```python
from build123d import *

# Parameters (mm, degrees)
ESQUISSE2_W                                      = 120
ESQUISSE2_H                                      = 90
BOSS_EXTRU_1_DEPTH                               = 2
ESQUISSE3_R                                      = 5
BOSS_EXTRU_2_DEPTH                               = 8
CHAMBRAGE_POUR_VIS_T_TE_RONDE_BOMB_E_D           = 3.7973
CHAMBRAGE_POUR_VIS_T_TE_RONDE_BOMB_E_CBORE_D     = 7.54126
CHAMBRAGE_POUR_VIS_T_TE_RONDE_BOMB_E_CBORE_DEPTH = 2.4638
R_P_TITION_LIN_AIRE1_COUNT                       = 2
R_P_TITION_LIN_AIRE1_PITCH                       = 96
R_P_TITION_LIN_AIRE1_COUNT_DIR2                  = 2
R_P_TITION_LIN_AIRE1_PITCH_DIR2                  = 66
ENL_V_MAT_EXTRU_1_DEPTH                          = 8
R_P_TITION_LIN_AIRE2_COUNT                       = 5
R_P_TITION_LIN_AIRE2_PITCH                       = 9
R_P_TITION_LIN_AIRE2_COL_COUNT                   = 5
R_P_TITION_LIN_AIRE2_COL_PITCH                   = 9
ESQUISSE8_W                                      = 120
ESQUISSE8_H                                      = 90
ESQUISSE8_W_2                                    = 116
ESQUISSE8_H_2                                    = 86
BOSS_EXTRU_3_DEPTH                               = 25
ENL_V_MAT_EXTRU_2_REACH                          = 132.973
ENL_V_MAT_EXTRU_3_DEPTH                          = 2
CONG_1_R                                         = 3


with BuildPart() as part:
    # Esquisse2 → Boss.-Extru.1 (new body)
    with BuildSketch(Plane.XY):
        Rectangle(ESQUISSE2_W, ESQUISSE2_H)
    extrude(amount=BOSS_EXTRU_1_DEPTH)

    # Esquisse3 → Boss.-Extru.2 (add)
    with BuildSketch(Plane.XY.offset(2)):
        with Locations((-48, 33)):
            Circle(ESQUISSE3_R)
        with Locations((48, 33)):
            Circle(ESQUISSE3_R)
        with Locations((48, -33)):
            Circle(ESQUISSE3_R)
        with Locations((-48, -33)):
            Circle(ESQUISSE3_R)
    extrude(amount=BOSS_EXTRU_2_DEPTH)

    # Chambrage pour vis à tête ronde bombée #61 (through all)
    with Locations(Plane(origin=(0, 0, 0), x_dir=(-1, 0, 0), z_dir=(0, 0, -1))):
        with Locations((48, -33)):
            chambrage_pour_vis_t_te_ronde_bomb_e = CounterBoreHole(CHAMBRAGE_POUR_VIS_T_TE_RONDE_BOMB_E_D / 2, CHAMBRAGE_POUR_VIS_T_TE_RONDE_BOMB_E_CBORE_D / 2, CHAMBRAGE_POUR_VIS_T_TE_RONDE_BOMB_E_CBORE_DEPTH)

    # Répétition linéaire1: Chambrage pour vis _ t_te ronde bomb_e 2 × 2
    with Locations(*[(i * R_P_TITION_LIN_AIRE1_PITCH, j * R_P_TITION_LIN_AIRE1_PITCH_DIR2, 0) for i in range(R_P_TITION_LIN_AIRE1_COUNT) for j in range(R_P_TITION_LIN_AIRE1_COUNT_DIR2) if (i, j) != (0, 0)]):
        add(chambrage_pour_vis_t_te_ronde_bomb_e, mode=Mode.SUBTRACT)

    # Esquisse7 → Enlèv. mat.-Extru.1 (cut)
    with BuildSketch(Plane.XY.offset(2)):
        with BuildLine():
            Line((-1.5, -30), (-1.5, 30))
            ThreePointArc((-1.5, 30), (0, 31.5), (1.5, 30))
            Line((1.5, 30), (1.5, -30))
            ThreePointArc((1.5, -30), (0, -31.5), (-1.5, -30))
        make_face()
    enl_v_mat_extru_1 = extrude(amount=-ENL_V_MAT_EXTRU_1_DEPTH, mode=Mode.SUBTRACT)

    # Répétition linéaire2: Enlèv. mat.-Extru.1 ×5
    with Locations(*[(-i * R_P_TITION_LIN_AIRE2_PITCH, 0, 0) for i in range(1, R_P_TITION_LIN_AIRE2_COUNT)]):
        add(enl_v_mat_extru_1, mode=Mode.SUBTRACT)

    # Répétition linéaire2 col: Enlèv. mat.-Extru.1 ×5
    with Locations(*[(i * R_P_TITION_LIN_AIRE2_COL_PITCH, 0, 0) for i in range(1, R_P_TITION_LIN_AIRE2_COL_COUNT)]):
        add(enl_v_mat_extru_1, mode=Mode.SUBTRACT)

    # Esquisse8 → Boss.-Extru.3 (add)
    with BuildSketch(Plane.XY.offset(2)):
        Rectangle(ESQUISSE8_W, ESQUISSE8_H)
        Rectangle(ESQUISSE8_W_2, ESQUISSE8_H_2, mode=Mode.SUBTRACT)
    extrude(amount=BOSS_EXTRU_3_DEPTH)

    # Esquisse9 → Enlèv. mat.-Extru.2 (cut, up to next)
    with BuildSketch(Plane.ZY.offset(60), mode=Mode.PRIVATE) as enl_v_mat_extru_2_sk1:
        with BuildLine():
            Line((23, 0.689181082), (23, -29.310818918))
            ThreePointArc((23, -29.310818918), (18, -34.310818918), (13, -29.310818918))
            Line((13, -29.310818918), (13, 0.689181082))
            ThreePointArc((13, 0.689181082), (18, 5.689181082), (23, 0.689181082))
        make_face()
    enl_v_mat_extru_2_tool1 = extrude(enl_v_mat_extru_2_sk1.sketch, amount=-ENL_V_MAT_EXTRU_2_REACH, mode=Mode.PRIVATE) & part.part
    add(enl_v_mat_extru_2_tool1.solids().sort_by_distance((-60, -14.310819, 18))[0], mode=Mode.SUBTRACT)

    # Esquisse10 → Enlèv. mat.-Extru.3 (cut)
    with BuildSketch(Plane(origin=(60, 0, 0), x_dir=(0, 0, -1), z_dir=(1, 0, 0))):
        with BuildLine():
            Line((-20, -8.249494847), (-20, 6.750505153))
            ThreePointArc((-20, 6.750505153), (-15, 11.750505153), (-10, 6.750505153))
            Line((-10, 6.750505153), (-10, -8.249494847))
            ThreePointArc((-10, -8.249494847), (-15, -13.249494847), (-20, -8.249494847))
        make_face()
    extrude(amount=-ENL_V_MAT_EXTRU_3_DEPTH, mode=Mode.SUBTRACT)

    # Congé1
    cong_1_edges = [part.edges().sort_by_distance(p)[0] for p in [
        (-60, 45, 13.5),
        (60, 45, 13.5),
        (60, -45, 13.5),
        (-60, -45, 13.5),
    ]]
    fillet(cong_1_edges, radius=CONG_1_R)


solid = part.part
```
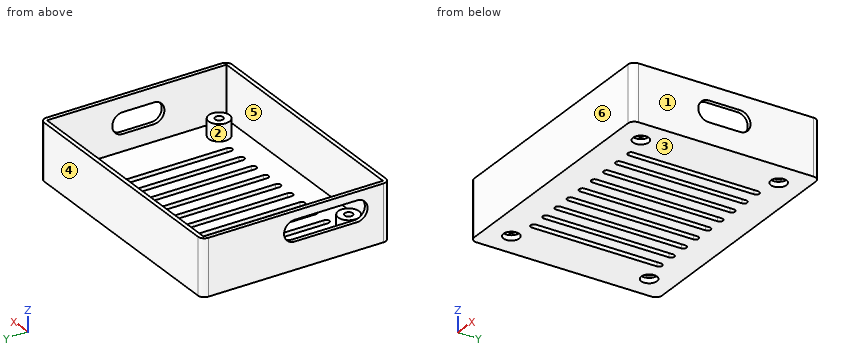
Design review of the part built by this model. Coordinates are the model's own, in mm. Face numbers are marked on the shaded views. A direction names the side the tool comes from. Give positions to 0.01 mm unless a question says otherwise; leave off trailing zeros. Write each loop counter-clockwise with the first axis right and the second up, starting at its lowest first coordinate (ties: lowest second). Pieces come first, ordered by that corner, then holes.
(1) Wall thickness on line 1 along Y through (x, z) = (-48, 0.6); line 2 along Y through (x, z) = (48, 4.75); line 3 along Y through (x, z) = (-6, 19.25): over which ranges is each line inside the solid? List them lowest first.
Checked values:
line 1: y = -45 to -36.77, -29.23 to 29.23, 36.77 to 45
line 2: y = -45 to -43, -38 to -34.9, -31.1 to -28, 28 to 31.1, 34.9 to 38, 43 to 45
line 3: y = -45 to -43, 43 to 45
(2) Tool access review of the marked faces 1 and 2: name each direction out of +Z, -Z, +X, -X, +Y, -Y from which nothing blocks a thin tool from reaching the whole face with its end or side.
Checked values:
face 1: +Z, -Z, +X, +Y, -Y
face 2: +Z
(3) Clearance check with flat-ended pins moving along their axes: pin 1 Ø1 at (x, y) = (22.5, 15) entering from -Z; pin 2 Ø1 at (x, y) = (-20, 13.5) entering from +Z; pin 3 Ø2.5 at (x, y) = (47, -31) entering from -Z; pin 4 Ø8 at (x, y) = (48, -34) entering from +Z. State where each tip first meets the part, or that it passes through.
Checked values:
pin 1: stops at z = 0
pin 2: stops at z = 2
pin 3: stops at z = 2.46
pin 4: stops at z = 10
(4) Add section A-A (z = 6.5). Give the number of separate pieces and of enclosed holes in the cut face, and give its area (3 significant figures).
Checked values:
separate pieces: 5
enclosed holes: 5
area: 1,090 mm2
(5) Mouldability with a two-part tool opening along Y and no side actions: class the marked faces 3, 4, 5 and 6 as +Y half, -Y half, draft (parallel to the pull), parting line (faces both ways), or undercut.
Checked values:
face 3: draft
face 4: +Y half
face 5: undercut
face 6: -Y half
(6) Add section C-C (x = -18). Give the boundary of the cut face in (y, z), and give its area (3 significant figures).
Checked values:
outline: (-45, 0) - (-31.5, 0) - (-31.5, 2) - (-43, 2) - (-43, 27) - (-45, 27) - close; (31.5, 0) - (45, 0) - (45, 27) - (43, 27) - (43, 2) - (31.5, 2) - close
area: 154 mm2
